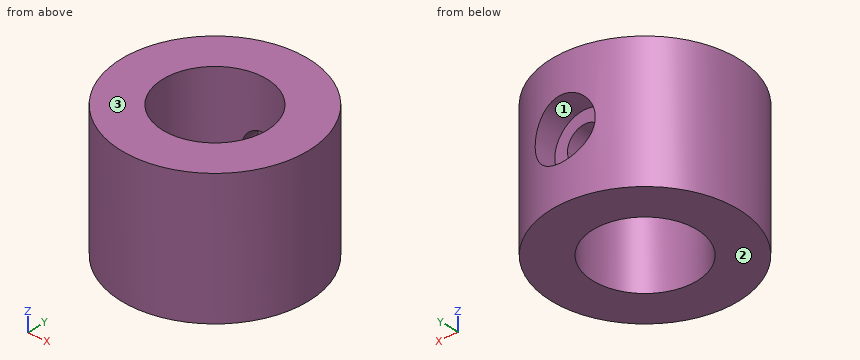
```python
from build123d import *

# Parameters (mm, degrees)
F0_R     = 8.89
F0_R_2   = 4.953
F1_DEPTH = 12.7
F3_DEPTH = 25.4
F5_R     = 2.8575
F6_DEPTH = 2.54


with BuildPart() as f1:
    # F0 (on Top) → F1 (new body)
    with BuildSketch(Plane.XY):
        Circle(F0_R)
        Circle(F0_R_2, mode=Mode.SUBTRACT)
    extrude(amount=F1_DEPTH)

    # F2 (on Front) → F3 (cut)
    with BuildSketch(Plane.XZ):
        with BuildLine():
            ThreePointArc((0, 4.699), (1.167433, 5.182567), (1.651, 6.35))
            ThreePointArc((1.651, 6.35), (-1.167433, 7.517433), (0, 4.699))
        make_face()
    extrude(amount=-F3_DEPTH, mode=Mode.SUBTRACT)

    # F5 (on offset) → F6 (cut)
    with BuildSketch(Plane.XZ.offset(-8.89)):
        with Locations((0, 6.35)):
            Circle(F5_R)
    extrude(amount=F6_DEPTH, mode=Mode.SUBTRACT)


solid = f1.part
```
The listing builds one solid part. Answer for the finished solid, in the listing's coordinates (mm). Face numbers are marked on the shaded views. Coordinates: 2 decimals unless noted, no trailing zeros. Write each loop counter-clockwise with the first axis right and the second up, starting at its lowest first coordinate (ties: lowest second). Pieces come first, ordered by that corner, then holes. Notation, with made-up numbers: (54, -23.75) - (113, -23.75) arc R31 ccw to (113, 8.25) - close; hole circle Ø9 at (-1.5, 15.25). An arc over 180 degrees is marked (long way). One line per item, written item: value.
1) Find section B-B (x = 1.25). Give the vertices of the cut face in (y, z), and give its area (3 significant figures).
Geometry check:
outline: (-8.8, 0) - (-4.79, 0) - (-4.79, 12.7) - (-8.8, 12.7) - close; (4.79, 0) - (8.8, 0) - (8.8, 3.78) - (6.35, 3.78) - (6.35, 5.27) - (4.79, 5.27) - close; (4.79, 7.43) - (6.35, 7.43) - (6.35, 8.92) - (8.8, 8.92) - (8.8, 12.7) - (4.79, 12.7) - close
area: 85.9 mm2
2) Find section C-C (z = 3.25). Give the vertices of the cut face in (x, y), and give its area (3 significant figures).
Geometry check:
outline: circle Ø17.78 at (0, 0); hole circle Ø9.91 at (0, 0)
area: 171 mm2
3) Find section A-A (y = 0). Give the vertices of the cut face in (x, z).
Geometry check:
outline: (-8.89, 0) - (-4.95, 0) - (-4.95, 12.7) - (-8.89, 12.7) - close; (4.95, 0) - (8.89, 0) - (8.89, 12.7) - (4.95, 12.7) - close
4) Consider line 1 along Z through (x, y) = (0, 7.55); line 2 along Y through (x, z) = (0, 8.5); line 3 along Y through (x, z) = (0, 10). Determine where each line is inside the solid, lowest interval first. Write a range as from..to.
Geometry check:
line 1: z = 0..3.49, 9.21..12.7
line 2: y = -8.89..-4.95, 4.95..6.35
line 3: y = -8.89..-4.95, 4.95..8.89
5) For a pull along Z with two mould halves and no side action, classify the marked faces 1, 2 and 3 as pulls with the +Z half, pulls with the -Z half, needs draft (parallel to the pull), parting line crosses it, or undercut.
Geometry check:
face 1: undercut
face 2: pulls with the -Z half
face 3: pulls with the +Z half
6) Each of these flat-tipped pins is pushed along its axis until it touches: pin 1 Ø1 at (y, z) = (-2.5, 11) entering from +X; pin 2 Ø1.7 at (x, z) = (0.5, 5) entering from +Y; pin 3 Ø3 at (y, z) = (-2.5, 5) entering from -X. Where does it stop, or does it pass through?
Geometry check:
pin 1: stops at x = 8.66
pin 2: stops at y = 6.35
pin 3: stops at x = -8.83
